from build123d import *


with BuildPart() as part:
    # Çizim1 → Döndür1 (revolve)
    with BuildSketch(Plane(origin=(0, 0, 0), x_dir=(0, 0, -1), z_dir=(1, 0, 0)), mode=Mode.PRIVATE) as d_nd_r1_sk:
        with BuildLine():
            Line((0, 7.25), (0, 60.706950554))
            Line((0, 60.706950554), (-4, 67))
            Line((-4, 67), (18.02567306, 81))
            Line((18.02567306, 81), (26, 68.454291568))
            Line((26, 68.454291568), (26, 54))
            ThreePointArc((26, 54), (28.928932188, 46.928932188), (36, 44))
            Line((36, 44), (46, 44))
            Line((46, 44), (46, 7.25))
            Line((46, 7.25), (0, 7.25))
        make_face()
    revolve(d_nd_r1_sk.sketch.rotate(Axis((0, 0, -100.24473813), (0, 0, 1)), 90), axis=Axis((0, 0, -100.24473813), (0, 0, 1)))


solid = part.part
Source: CAD feature listing. Evaluate the final solid. Frame: model axes, mm. A direction names the side the tool comes from. Round coordinates to 2 decimals unless told otherwise and drop trailing zeros. Loops run counter-clockwise (first coordinate to the right, second up) from the corner with the lowest first, then second, coordinate; pieces in that order, holes last.
Q1. Section D-D, the plane z = -43. Return loops of the section in (x, y).
Q2. First-contact query: P1, Ø10, axis at x = -54, z = -3, coming from the +Y side; P2, Ø3, axis at x = -49, z = -26, coming from the +Y side; P3, Ø2, axis at x = -34, z = -36.5, coming from the -Y side. Flat tips, straight axial feed; report the tip coordinate or a pass-through.
Q3. Mould query, pull axis X, two halves, no side actions, for faces 1 (the face through (-58.28, -18.35, 0.25)), 2 (the face through (9.538, 42.954, -41.07)), 3 (the face through (-50, -21, -26)). Classes: pulls with the +X half, pulls with the -X half, needs draft (parallel to the pull), parting line crosses it, or undercut.
Q4. Ray query, line 1 (Z direction, x = 20, y = 50); line 2 (Y direction, x = -18.5, z = 1); line 3 (Z direction, x = 2, y = 13.5). Return the intervals inside material, ascending.
Q5. Access query for faces 4 (the face through (-1, 13, 0)), 5 (the face through (8.99, -68.48, -25.61)). Directions: +Z, -Z, +X, -X, +Y, -Y. A direction counts if a zero-diameter tool reaches every point of the face in a straight line with its end or side. Return the directions, or none.
Q6. Section A-A, the plane x = 0. Return loops of the section in (y, z), plus the area to 3 significant figures.
Q7. Section C-C, the plane z = -28. Return loops of the section in (x, y).
Solutions:
1. outline: circle Ø88 at (0, 0); hole circle Ø14.5 at (0, 0)
2. P1: stops at y = 53.71
2. P2: stops at y = 51.42
2. P3: stops at y = -29.1
3. face 1: undercut
3. face 2: parting line crosses it
3. face 3: needs draft
4. line 1: z = -26 to 0
4. line 2: y = -66.38 to -59.47, 59.47 to 66.38
4. line 3: z = -46 to 0
5. face 4: +Z
5. face 5: -Z
6. outline: (-81, -18.03) - (-68.45, -26) - (-54, -26) arc R10 cw to (-44, -36) - (-44, -46) - (-7.25, -46) - (-7.25, 0) - (-60.71, 0) - (-67, 4) - close; (7.25, -46) - (44, -46) - (44, -36) arc R10 cw to (54, -26) - (68.45, -26) - (81, -18.03) - (67, 4) - (60.71, 0) - (7.25, 0) - close
6. area: 5,080 mm2
7. outline: circle Ø96 at (0, 0); hole circle Ø14.5 at (0, 0)
